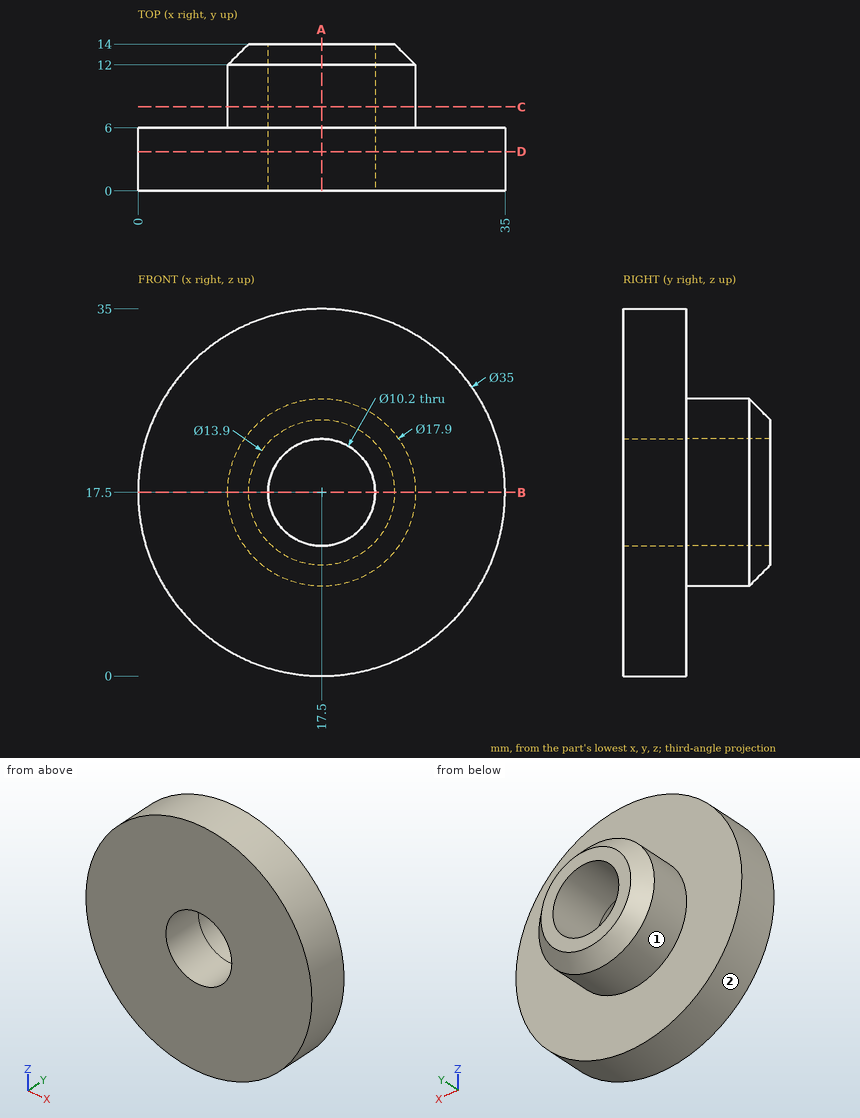
Study the drawing (mm; zero at the part's minimum x, y, z) and answer. A direction names the side the tool comes from. Coordinates: 2 decimals unless noted, no trailing zeros. Write each loop counter-clockwise with the first axis right and the second up, starting at its lowest first coordinate (ties: lowest second). Pieces come first, ordered by that corner, then holes. Notation, with made-up numbers: (-33.75, -13) - (23.25, -13) arc R23 ccw to (23.25, 21) - close; hole circle Ø7 at (81, -26.5). An arc over 180 degrees is marked (long way). Answer as a JSON object with one key per item and string values. Group by question number.
1. A cutting plane is placed at C-C (y = 8). Determine the outline of the cut face in (x, z).
2. Consider L1, parallel to Z at x = 17.5, y = 3.55; L2, parallel to Z at x = 17.5, y = 8.25; L3, parallel to Y at x = 4.5, z = 15.5. Determine where each line is inside the solid, lowest interval first. Write a range as [from, to].
3. A cutting plane is placed at D-D (y = 3.75). Determine the outline of the cut face in (x, z), plus the area to 3 significant figures.
4. Each of these flat-tipped pins is pushed along its axis until it touches: P1, Ø1.5, axis at y = 11.5, z = 8.5, coming from the +X side; P2, Ø6, axis at y = 7.5, z = 24, coming from the +X side; P3, Ø16.5, axis at x = 17.5, z = 17.5, coming from the -Y side; P4, Ø1.5, axis at y = 3, z = 13.5, coming from the +X side. Where does it stop, or does it pass through?
5. A cutting plane is placed at B-B (z = 17.5). Determine the outline of the cut face in (x, y).
6. A cutting plane is placed at A-A (x = 17.5). Determine the outline of the cut face in (y, z), plus the area to 3 significant figures.
7. Which of the six approach directions +Z, -Z, +X, -X, +Y, -Y give full straight-line access (tool end or side, diameter ignored) to the marked faces 1 and 2?
Worked out:
{
 "1": {"outline": "circle Ø17.9 at (17.5, 17.5); hole circle Ø10.2 at (17.5, 17.5)"},
 "2": {"L1": "z = [0, 12.4], [22.6, 35]", "L2": "z = [8.55, 12.4], [22.6, 26.45]", "L3": "y = [0, 6]"},
 "3": {"outline": "circle Ø35 at (17.5, 17.5); hole circle Ø10.2 at (17.5, 17.5)", "area": "880 mm²"},
 "4": {"P1": "stops at x = 20.97", "P2": "stops at x = 34.56", "P3": "stops at y = 0", "P4": "stops at x = 34.7"},
 "5": {"outline": "(0, 0) - (12.4, 0) - (12.4, 14) - (10.55, 14) - (8.55, 12) - (8.55, 6) - (0, 6) - close; (22.6, 0) - (35, 0) - (35, 6) - (26.45, 6) - (26.45, 12) - (24.45, 14) - (22.6, 14) - close"},
 "6": {"outline": "(0, 0) - (6, 0) - (6, 8.55) - (12, 8.55) - (14, 10.55) - (14, 12.4) - (0, 12.4) - close; (0, 22.6) - (14, 22.6) - (14, 24.45) - (12, 26.45) - (6, 26.45) - (6, 35) - (0, 35) - close", "area": "206 mm²"},
 "7": {"face 1": "+Y", "face 2": "+Y, -Y"}
}
